Design review of the part built by this model. Coordinates are the model's own, in mm. A direction names the side the tool comes from. Round coordinates to 2 decimals unless told otherwise and drop trailing zeros. Loops run counter-clockwise (first coordinate to the right, second up) from the corner with the lowest first, then second, coordinate; pieces in that order, holes last. Notation, with made-up numbers: M 37,12.25 L 46,12.25 A24 cw 46,22.25 Z; hole C -28,-10 d3. An arc over 180 degrees is marked long. Answer as CSV lines item,"result". Start each with the question number.
from build123d import *

# Parameters (mm, degrees)
F0_R     = 0.625
F0_W     = 24
F0_H     = 13.5
F0_R_2   = 1.25
F1_DEPTH = 3
F3_R     = 3


with BuildPart() as f1:
    # F0 (on Top) → F1 (new body)
    with BuildSketch(Plane.XY):
        Polygon((20, -12.5), (20, 12.5), (16, 12.5), (-20, 12.5), (-20, -12.5), align=None)
        with Locations((-13.75, -5)):
            Circle(F0_R, mode=Mode.SUBTRACT)
        with Locations((0, -5)):
            Rectangle(F0_W, F0_H, mode=Mode.SUBTRACT)
        with Locations((13.75, -5)):
            Circle(F0_R, mode=Mode.SUBTRACT)
        with Locations((-16, 8.5)):
            Circle(F0_R_2, mode=Mode.SUBTRACT)
        with Locations((16, 8.5)):
            Circle(F0_R_2, mode=Mode.SUBTRACT)
    extrude(amount=F1_DEPTH)

    # F2: F1 across face


with BuildPart() as f1_1:
    add(f1.part)
    add(f1.part.mirror(Plane(origin=(0, -12.5, 1.5), x_dir=(1, 0, 0), z_dir=(0, -1, 0))))

    # F3
    f3_edges = [f1_1.edges().sort_by_distance(p)[0] for p in [
        (-20, -37.5, 1.5),
        (20, -37.5, 1.5),
        (20, 12.5, 1.5),
        (-20, 12.5, 1.5),
    ]]
    fillet(f3_edges, radius=F3_R)


solid = f1_1.part
Item 1: To check wall thickness, follow line 1 (Y direction, x = 1, z = 2.2); line 2 (Y direction, x = -13.75, z = 1.55) (3 decimals); line 3 (X direction, y = -20, z = 2.4) (3 decimals). State the ranges of each line that lie inside material, in increasing order.
Item 2: Consider section B-B, the plane x = -13.75. Write out the cut boundary in (y, z) (3 decimals).
Item 3: Tool access review of faces 1 (the face through (0, -13, 0)), 2 (the face through (0, -26.75, 1)): name each direction out of +Z, -Z, +X, -X, +Y, -Y from which nothing blocks a thin tool from reaching the whole face with its end or side.
Item 4: The part is to be moulded in two halves that separate along X. For faces 3 (the face through (0, -13.25, 1)), 4 (the face through (15.73, -32.28, 1.48)), 5 (the face through (0, -37.5, 1)), 6 (the face through (-19.14, 11.6, 1.52)), say which applies: +X half, -X half, draft (parallel to the pull), parting line (faces both ways), or undercut.
Item 5: Insertion check: pin 1 Ø1.1 at (x, y) = (13.75, -20) entering from -Z. The pin has a flat end and moves straight along its axis. Give the tip position at first contact, or say it passes through.
Item 6: Consider section C-C, the plane z = 0.7. Count the separate pieces of the cut face and the enclosed holes in it, then the cut area to 3 significant figures.
Item 7: Consider section A-A, the plane y = -20. Write out the cut boundary in (x, z) (3 decimals), then the cut area to 3 significant figures.
Item 8: Consider section D-D, the plane y = 0.5. Write out the cut boundary in (x, z), then the cut area to 3 significant figures.
Found:
1,line 1,"y = -37.5 to -26.75, -13.25 to -11.75, 1.75 to 12.5"
1,line 2,"y = -37.5 to -20.625, -19.375 to -5.625, -4.375 to 12.5"
1,line 3,"x = -20 to -14.375, -13.125 to -12, 12 to 13.125, 14.375 to 20"
2,outline,"M -37.5,0 L -20.625,0 L -20.625,3 L -37.5,3 Z; M -19.375,0 L -5.625,0 L -5.625,3 L -19.375,3 Z; M -4.375,0 L 12.5,0 L 12.5,3 L -4.375,3 Z"
3,face 1,"-Z, +X, -X, +Y, -Y"
3,face 2,"+Z, -Z"
4,face 3,"undercut"
4,face 4,"undercut"
4,face 5,"draft"
4,face 6,"-X half"
5,pin 1,"passes through"
6,separate pieces,"1"
6,enclosed holes,"10"
6,area,"1,320 mm^2"
7,outline,"M -20,0 L -14.375,0 L -14.375,3 L -20,3 Z; M -13.125,0 L -12,0 L -12,3 L -13.125,3 Z; M 12,0 L 13.125,0 L 13.125,3 L 12,3 Z; M 14.375,0 L 20,0 L 20,3 L 14.375,3 Z"
7,area,"40.5 mm^2"
8,outline,"M -20,0 L -12,0 L -12,3 L -20,3 Z; M 12,0 L 20,0 L 20,3 L 12,3 Z"
8,area,"48.0 mm^2"
